Part model, mm, in its own coordinate system. A direction names the side the tool comes from. Give positions to 0.01 mm unless a question says otherwise; leave off trailing zeros. Order: outer loops, then holes, each group sorted by start corner. A loop starts at its lowest first (then second) coordinate and runs counter-clockwise, first axis right, second up. Notation, with made-up numbers: M 48.5,33 L 102.5,33 A32 ccw 102.5,69 Z; hole C 65,60.25 d5. An arc over 180 degrees is marked long. Answer as a JSON object with one key per item and string values.
from build123d import *

# Parameters (mm, degrees)
BOSS_EXTRU_1_DEPTH                                 = 18
ESQUISSE2_W                                        = 11
ESQUISSE2_H                                        = 19
ENL_V_MAT_EXTRU_1_DEPTH                            = 33
CHAMBRAGE_POUR_VIS_T_TE_HEXAGONALE_M41_D           = 4.5
CHAMBRAGE_POUR_VIS_T_TE_HEXAGONALE_M41_CBORE_D     = 8
CHAMBRAGE_POUR_VIS_T_TE_HEXAGONALE_M41_CBORE_DEPTH = 4.4
CHAMBRAGE_POUR_VIS_T_TE_HEXAGONALE_M44_D           = 4.5
CHAMBRAGE_POUR_VIS_T_TE_HEXAGONALE_M44_CBORE_D     = 9
CHAMBRAGE_POUR_VIS_T_TE_HEXAGONALE_M44_CBORE_DEPTH = 3
ESQUISSE9_R                                        = 5.5
ENL_V_MAT_EXTRU_2_DEPTH                            = 8
ESQUISSE10_R                                       = 7
ENL_V_MAT_EXTRU_3_DEPTH                            = 5
ESQUISSE11_W                                       = 9
ESQUISSE11_H                                       = 6
ENL_V_MAT_EXTRU_4_DEPTH                            = 8
CHANFREIN1_SIZE                                    = 17
CONG_1_R                                           = 5
CONG_2_R                                           = 5


with BuildPart() as part:
    # Esquisse1 → Boss.-Extru.1 (new body)
    with BuildSketch(Plane(origin=(0, 0, 0), x_dir=(0, 0, -1), z_dir=(1, 0, 0))):
        Polygon((0, 0), (5.642463383, 32), (28, 32), (28, 0), align=None)
    extrude(amount=BOSS_EXTRU_1_DEPTH)

    # Esquisse2 → Enlèv. mat.-Extru.1 (cut, through all)
    with BuildSketch(Plane(origin=(0, 32, 0), x_dir=(1, 0, 0), z_dir=(0, 1, 0))):
        with Locations((12.5, 18.5)):
            Rectangle(ESQUISSE2_W, ESQUISSE2_H)
    extrude(amount=-ENL_V_MAT_EXTRU_1_DEPTH, mode=Mode.SUBTRACT)

    # Chambrage pour vis à tête hexagonale M41 (through all)
    with Locations(Plane(origin=(0, 0, -9), x_dir=(-1, 0, 0), z_dir=(0, 0, -1))):
        with Locations((-12.5, 6)):
            CounterBoreHole(CHAMBRAGE_POUR_VIS_T_TE_HEXAGONALE_M41_D / 2, CHAMBRAGE_POUR_VIS_T_TE_HEXAGONALE_M41_CBORE_D / 2, CHAMBRAGE_POUR_VIS_T_TE_HEXAGONALE_M41_CBORE_DEPTH)

    # Chambrage pour vis à tête hexagonale M44 (through all)
    with Locations(Plane(origin=(0, 0, -9), x_dir=(-1, 0, 0), z_dir=(0, 0, -1))):
        with Locations((-12.5, 25.5)):
            CounterBoreHole(CHAMBRAGE_POUR_VIS_T_TE_HEXAGONALE_M44_D / 2, CHAMBRAGE_POUR_VIS_T_TE_HEXAGONALE_M44_CBORE_D / 2, CHAMBRAGE_POUR_VIS_T_TE_HEXAGONALE_M44_CBORE_DEPTH)

    # Esquisse9 → Enlèv. mat.-Extru.2 (cut, through all)
    with BuildSketch(Plane(origin=(7, 0, 0), x_dir=(0, 0, -1), z_dir=(1, 0, 0))):
        with Locations((19, 23)):
            Circle(ESQUISSE9_R)
    extrude(amount=-ENL_V_MAT_EXTRU_2_DEPTH, mode=Mode.SUBTRACT)

    # Esquisse10 → Enlèv. mat.-Extru.3 (cut)
    with BuildSketch(Plane(origin=(7, 0, 0), x_dir=(0, 0, -1), z_dir=(1, 0, 0))):
        with Locations((19, 23)):
            Circle(ESQUISSE10_R)
    extrude(amount=-ENL_V_MAT_EXTRU_3_DEPTH, mode=Mode.SUBTRACT)

    # Esquisse11 → Enlèv. mat.-Extru.4 (cut, through all)
    with BuildSketch(Plane(origin=(7, 0, 0), x_dir=(0, 0, -1), z_dir=(1, 0, 0))):
        with Locations((23.5, 23)):
            Rectangle(ESQUISSE11_W, ESQUISSE11_H)
    extrude(amount=-ENL_V_MAT_EXTRU_4_DEPTH, mode=Mode.SUBTRACT)

    # Chanfrein1
    chanfrein1_edges = [part.edges().sort_by_distance(p)[0] for p in [
        (3.5, 0, -28),
    ]]
    chamfer(chanfrein1_edges, length=CHANFREIN1_SIZE)

    # Congé1
    cong_1_edges = [part.edges().sort_by_distance(p)[0] for p in [
        (3.5, 32, -28),
    ]]
    fillet(cong_1_edges, radius=CONG_1_R)

    # Congé2
    cong_2_edges = [part.edges().sort_by_distance(p)[0] for p in [
        (18, 32, -7.321231691),
        (18, 0, -4.5),
    ]]
    fillet(cong_2_edges, radius=CONG_2_R)


solid = part.part
1. Cut at D-D on x = 12.5. Give the cut face in (y, z), plus the area to 3 significant figures.
Worked answers:
{"outline": "M 0,-9 L 2,-9 L 2,-4.6 L 3.75,-4.6 L 3.75,-0.66 L 0,0 Z; M 8.25,-4.6 L 10,-4.6 L 10,-9 L 21,-9 L 21,-6 L 23.25,-6 L 23.25,-4.1 L 8.25,-1.45 Z; M 27.75,-6 L 30,-6 L 30,-9 L 32,-9 L 32,-5.64 L 27.75,-4.89 Z", "area": "113 mm^2"}
2. Probe line 1 along Y through (x, z) = (3, -27); line 2 along Y through (x, z) = (5.7, -19); line 3 along X through (y, z) = (30, -23.5). List the from-to ranges inside material, lowest first.
Worked answers:
{"line 1": "y = 16 to 20, 26 to 30", "line 2": "y = 8 to 16, 30 to 32", "line 3": "x = 0 to 7"}
3. Cut at A-A on z = -19. Give the cut face in (x, y).
Worked answers:
{"outline": "M 0,8 L 7,8 L 7,16 L 2,16 L 2,17.5 L 0,17.5 Z; M 0,28.5 L 2,28.5 L 2,30 L 7,30 L 7,32 L 0,32 Z"}
4. Two-plate mould, pull along Z, no slides. Class faces 5 (the flat face through (0, 16, -11)), 6 (the cylindrical face through (1.014, 23.197, -13.504)), 7 (the flat face through (3, 19, -28)): +Z half, -Z half, draft (parallel to the pull), parting line (faces both ways), or undercut.
Worked answers:
{"face 5": "draft", "face 6": "undercut", "face 7": "-Z half"}
5. Cut at B-B on z = -7.5. Give the cut face in (x, y), plus the area to 3 significant figures.
Worked answers:
{"outline": "M 0,0 L 13,0 A5 ccw 18,5 L 18,27 A5 ccw 13,32 L 0,32 Z; hole C 12.5,25.5 d9; hole C 12.5,6 d8", "area": "451 mm^2"}
6. Pin check, flat tips, straight feed: P1, Ø1, axis at x = 4.5, y = 8, coming from the -Z side; P2, Ø5.5, axis at y = 10.5, z = -14.5, coming from the +X side; P3, Ø2, axis at x = 3.5, z = -26, coming from the -Y side; P4, Ø3.5, axis at x = 12.5, y = 25.5, coming from the +Z side. Stop position of each tip, or through.
Worked answers:
{"P1": "stops at z = -19.5", "P2": "stops at x = 7", "P3": "stops at y = 14", "P4": "passes through"}
7. Which spindle directions (+Z, -Z, +X, -X, +Y, -Y) get a long thin tool onto all of the face, cutting with end or side? Do faces 1 (the flat face through (2, 21, -13.7)), 2 (the flat face through (3, 26, -26)), 3 (the flat face through (12, 28, -6)), 4 (the flat face through (7, 16, -16)). Say none if no direction does.
Worked answers:
{"face 1": "+X", "face 2": "-Z, +X, -X", "face 3": "-Z", "face 4": "-Z, +X, +Y, -Y"}
8. Cut at C-C on y = 4.5. Give the cut face in (x, z), plus the area to 3 significant figures.
Worked answers:
{"outline": "M 0,-15.5 L 7,-15.5 L 7,-9 L 8.79,-9 L 8.79,-4.6 L 10.82,-4.6 L 10.82,-0.79 L 0,-0.79 Z; M 14.18,-4.6 L 16.21,-4.6 L 16.21,-9 L 17.97,-9 L 17.97,-0.79 L 14.18,-0.79 Z", "area": "148 mm^2"}
